```python
from build123d import *

# Parameters (mm, degrees)
F0_W     = 31.75
F0_H     = 31.75
F1_DEPTH = 120.65
F3_DEPTH = 5.08


with BuildPart() as f1:
    # F0 (on Top) → F1 (new body, symmetric)
    with BuildSketch(Plane.XY):
        Rectangle(F0_W, F0_H)
    extrude(amount=F1_DEPTH, both=True)

    # F2 (on face) → F3 (cut)
    with BuildSketch(Plane(origin=(-15.875, 0, 0), x_dir=(0, -1, 0), z_dir=(-1, 0, 0))):
        Polygon((15.875, 0), (15.875, 1.5875), (8.69188, 1.5875), (8.69188, 0), (8.69188, -1.5875), (15.875, -1.5875), align=None)
    extrude(amount=-F3_DEPTH, mode=Mode.SUBTRACT)


solid = f1.part
```
The listing builds one solid part. Answer for the finished solid, in the listing's coordinates (mm). Give positions to 0.01 mm unless a question says otherwise; leave off trailing zeros. Write each question's results on one line, items separated by ' | '.
Q1. A straight line is drawn through the part: probe 1 along Z at (x, y) = (-14, -9). Find the intervals that lie inside material, in ascending order. Write a range as from..to.
Checked values:
probe 1: z = -120.65..-1.59, 1.59..120.65
Q2. Determine the mould class of faces 1 (the face through (-13, -12, -1.588)), 2 (the face through (-13, -12, 1.588)), 3 (the face through (0, 0, 120.65)), 4 (the face through (15.875, 0, 2)) for opening direction Z: pulls with the +Z half, pulls with the -Z half, needs draft (parallel to the pull), parting line crosses it, or undercut.
Checked values:
face 1: undercut | face 2: undercut | face 3: pulls with the +Z half | face 4: needs draft
Q3. This flat-tipped pin is pushed along its axis until it touches: P1, Ø1.6, axis at x = -14.5, z = 0.5, coming from the -Y side. Where does it stop, or does it pass through?
Checked values:
P1: stops at y = -8.69
